Input: part model. Units: mm. Frame: model coordinates. Round coordinates to 2 decimals unless told otherwise and drop trailing zeros. Order: outer loops, then holes, each group sorted by start corner. A loop starts at its lowest first (then second) coordinate and runs counter-clockwise, first axis right, second up. Notation, with made-up numbers: (14, -17) -> (19, -17) arc R25 ccw to (19, -4) -> close; hole circle Ø11 at (85, 23.25). An arc over 180 degrees is marked (long way). Use a Markdown table: item, result.
from build123d import *

# Parameters (mm, degrees)
F0_W     = 100
F0_H     = 40
F1_DEPTH = 3
F3_DEPTH = 25
F4_R     = 3


with BuildPart() as f1:
    # F0 (on Front) → F1 (new body)
    with BuildSketch(Plane.XZ):
        Rectangle(F0_W, F0_H)
    extrude(amount=F1_DEPTH)

    # F2 (on face) → F3 (cut)
    with BuildSketch(Plane.XZ.offset(3)):
        with BuildLine():
            ThreePointArc((39.5, -4.5), (44, 0), (39.5, 4.5))
            Line((39.5, 4.5), (30.5, 4.5))
            ThreePointArc((30.5, 4.5), (26, 0), (30.5, -4.5))
            Line((30.5, -4.5), (39.5, -4.5))
        make_face()
        with BuildLine():
            ThreePointArc((-39.5, 4.5), (-44, 0), (-39.5, -4.5))
            Line((-39.5, -4.5), (-30.5, -4.5))
            ThreePointArc((-30.5, -4.5), (-26, 0), (-30.5, 4.5))
            Line((-30.5, 4.5), (-39.5, 4.5))
        make_face()
    extrude(amount=-F3_DEPTH, mode=Mode.SUBTRACT)

    # F4
    f4_edges = [f1.edges().sort_by_distance(p)[0] for p in [
        (50, -1.5, -20),
        (50, -1.5, 20),
        (-50, -1.5, 20),
        (-50, -1.5, -20),
    ]]
    fillet(f4_edges, radius=F4_R)


solid = f1.part
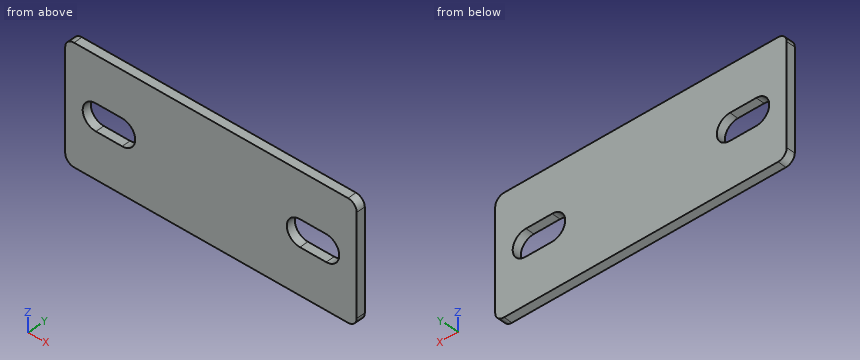
1) Pin query (flat end, axial travel): pin 1 Ø2 at (x, z) = (29.5, -1.5) entering from +Y. Return the tip coordinate at first contact, or that it passes through.
Results found:
| item | result |
|---|---|
| pin 1 | passes through |
2) Cut plane C-C on y = -0.6. Return loops of the section in (x, z), and give its area (3 significant figures).
Results found:
| item | result |
|---|---|
| outline | (-50, -17) arc R3 ccw to (-47, -20) -> (47, -20) arc R3 ccw to (50, -17) -> (50, 17) arc R3 ccw to (47, 20) -> (-47, 20) arc R3 ccw to (-50, 17) -> close; hole (-39.5, -4.5) -> (-30.5, -4.5) arc R4.5 ccw to (-30.5, 4.5) -> (-39.5, 4.5) arc R4.5 ccw to start; hole (30.5, -4.5) -> (39.5, -4.5) arc R4.5 ccw to (39.5, 4.5) -> (30.5, 4.5) arc R4.5 ccw to start |
| area | 3,700 mm² |
3) Line query: L1, parallel to Z at x = -36.5, y = -1.75; L2, parallel to X at y = -0.15, z = -1; L3, parallel to X at y = -1.5, z = -1.5. Output: solid intervals per line, ascending. Write a range as [from, to].
Results found:
| item | result |
|---|---|
| L1 | z = [-20, -4.5], [4.5, 20] |
| L2 | x = [-50, -43.89], [-26.11, 26.11], [43.89, 50] |
| L3 | x = [-50, -43.74], [-26.26, 26.26], [43.74, 50] |
4) Cut plane B-B on x = -27.5. Return loops of the section in (y, z).
Results found:
| item | result |
|---|---|
| outline | (-3, -20) -> (0, -20) -> (0, -3.35) -> (-3, -3.35) -> close; (-3, 3.35) -> (0, 3.35) -> (0, 20) -> (-3, 20) -> close |
5) Cut plane A-A on z = 0. Return loops of the section in (x, y).
Results found:
| item | result |
|---|---|
| outline | (-50, -3) -> (-44, -3) -> (-44, 0) -> (-50, 0) -> close; (-26, -3) -> (26, -3) -> (26, 0) -> (-26, 0) -> close; (44, -3) -> (50, -3) -> (50, 0) -> (44, 0) -> close |
